```python
from build123d import *

# Parameters (mm, degrees)
SKETCH001_W  = 28
SKETCH001_H  = 5
PAD001_DEPTH = 15
SKETCH002_W  = 1
SKETCH002_H  = 2
POCKET_DEPTH = 2
CHAMFER_SIZE = 1.99
FILLET_R     = 1
FILLET001_R  = 0.25
FILLET002_R  = 0.25


with BuildPart() as part:
    # Sketch001 → Pad001 (new body)
    with BuildSketch(Plane(origin=(-3.75, 0.6, 1.3), x_dir=(1, 0, 0), z_dir=(0, 1, 0))):
        with Locations((12.9, -1.2)):
            Rectangle(SKETCH001_W, SKETCH001_H)
    extrude(amount=PAD001_DEPTH)

    # Sketch002 → Pocket (cut)
    with BuildSketch(Plane(origin=(-3.75, 15.6, 1.3), x_dir=(1, 0, 0), z_dir=(0, 1, 0))):
        with Locations((18.6, -2.7)):
            Rectangle(SKETCH002_W, SKETCH002_H)
        with Locations((20.6, -2.7)):
            Rectangle(SKETCH002_W, SKETCH002_H)
    extrude(amount=-POCKET_DEPTH, mode=Mode.SUBTRACT)

    # Chamfer
    chamfer_edges = [part.edges().sort_by_distance(p)[0] for p in [
        (16.85, 13.6, 3),
        (14.85, 13.6, 3),
    ]]
    chamfer(chamfer_edges, length=CHAMFER_SIZE)

    # Fillet
    fillet_edges = [part.edges().sort_by_distance(p)[0] for p in [
        (-4.85, 15.6, 2.5),
        (23.15, 15.6, 2.5),
    ]]
    fillet(fillet_edges, radius=FILLET_R)

    # Fillet001
    fillet001_edges = [part.edges().sort_by_distance(p)[0] for p in [
        (-4.85, 7.6, 0),
        (-4.557107, 15.307107, 0),
        (9.15, 0.6, 0),
        (9.15, 15.6, 0),
        (23.15, 7.6, 0),
        (22.857107, 15.307107, 0),
    ]]
    fillet(fillet001_edges, radius=FILLET001_R)

    # Fillet002
    fillet002_edges = [part.edges().sort_by_distance(p)[0] for p in [
        (22.857107, 15.307107, 5),
        (23.15, 7.6, 5),
        (19.75, 15.6, 5),
        (15.85, 15.6, 5),
        (5.25, 15.6, 5),
        (-4.557107, 15.307107, 5),
        (-4.85, 7.6, 5),
    ]]
    fillet(fillet002_edges, radius=FILLET002_R)


solid = part.part
```
Geometry check sheet. Reference: the model listing, model coordinates, mm. A direction names the side the tool comes from. Coordinates: 2 decimals unless noted, no trailing zeros. Use one line per item in the form item = value. Start each with the question number.
1) Set-up check for faces 4 (the flat face through (14.35, 15, 4)), 5 (the flat face through (9, 8, 0)): record each of +Z, -Z, +X, -X, +Y, -Y from which the full face is reachable in a straight line by a thin tool's end or side.
2) Go/stop test with flat-tipped pins: pin 1 Ø0.6 at (y, z) = (15, 4.5) entering from -X (3 decimals); pin 2 Ø1.6 at (y, z) = (15, 4.5) entering from +X. Record where each tip stops, or that it passes through.
3) Thickness scan on probe 1 along X at (y, z) = (3, 0.2); probe 2 along Z at (x, y) = (14.5, 14); probe 3 along Y at (x, z) = (14.5, 4.1). Record the ranges inside material, lowest first. Write a range as from..to.
4) Release check for a two-part mould opening along X. For faces 1 (the flat face through (9, 15.6, 2)), 2 (the flat face through (23.15, 8, 3)), 3 (the flat face through (16.35, 15, 4)) record: pulls with the +X half, pulls with the -X half, needs draft (parallel to the pull), parting line crosses it, or undercut.
Responses:
q1.face_4 = +Z, +Y
q1.face_5 = -Z, +X, -X, +Y, -Y
q2.pin_1 = -4.845
q2.pin_2 = 23.15
q3.probe_1 = -4.84..23.14
q3.probe_2 = 0..4.59
q3.probe_3 = 0.6..14.49
q4.face_1 = needs draft
q4.face_2 = pulls with the +X half
q4.face_3 = undercut
